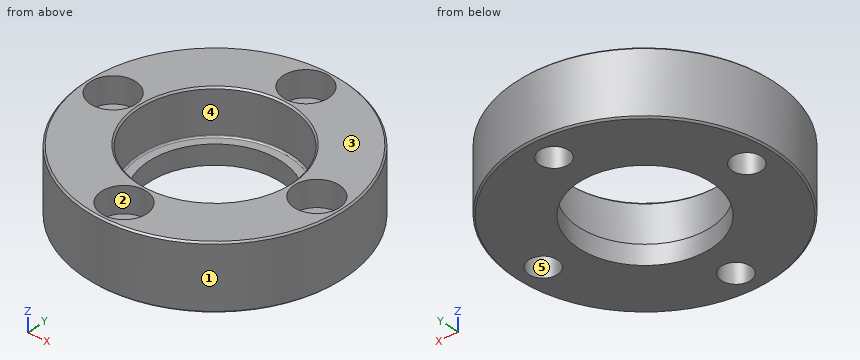
from build123d import *

# Parameters (mm, degrees)
F0_R           = 40
F0_R_2         = 20.5
F1_DEPTH       = 10
F2_R           = 23.5
F3_DEPTH       = 14
F4_R           = 0.5
F5_SIZE        = 0.5
F7_D           = 9
F7_CBORE_D     = 14
F7_CBORE_DEPTH = 8


with BuildPart() as f1:
    # F0 (on Top) → F1 (new body, symmetric)
    with BuildSketch(Plane.XY):
        Circle(F0_R)
        Circle(F0_R_2, mode=Mode.SUBTRACT)
    extrude(amount=F1_DEPTH, both=True)

    # F2 (on face) → F3 (cut)
    with BuildSketch(Plane.XY.offset(10)):
        Circle(F2_R)
    extrude(amount=-F3_DEPTH, mode=Mode.SUBTRACT)

    # F4
    f4_edges = [f1.edges().sort_by_distance(p)[0] for p in [
        (-23.5, 0, -4),
    ]]
    fillet(f4_edges, radius=F4_R)

    # F5
    f5_edges = [f1.edges().sort_by_distance(p)[0] for p in [
        (-23.5, 0, 10),
        (-40, 0, 10),
        (-40, 0, -10),
    ]]
    chamfer(f5_edges, length=F5_SIZE)

    # F7 (through all)
    with Locations(Plane.XY.offset(10)):
        with Locations((0, 31.75), (0, -31.75), (31.75, 0), (-31.75, 0)):
            CounterBoreHole(F7_D / 2, F7_CBORE_D / 2, F7_CBORE_DEPTH)


solid = f1.part
Geometry: final body of the model. Coordinates: model frame, mm. Face numbers are marked on the shaded views. A direction names the side the tool comes from. Round coordinates to 2 decimals unless told otherwise and drop trailing zeros. Order: outer loops, then holes, each group sorted by start corner. A loop starts at its lowest first (then second) coordinate and runs counter-clockwise, first axis right, second up. Notation, with made-up numbers: (55, 7.5) -> (98, 7.5) arc R19 ccw to (98, 24.5) -> close; hole circle Ø7 at (87.25, 7). An arc over 180 degrees is marked (long way). Put each result on its own line as item: value. Start each with the question number.
Q1. First-contact query: pin 1 (11 mm diameter, centred on x = -32, y = 2, fed in from +Z); pin 2 (6 mm diameter, centred on y = 10.5, z = 5.5, fed in from -X); pin 3 (6 mm diameter, centred on x = 24, z = 7, fed in from +Y); pin 4 (7 mm diameter, centred on x = -3, y = -33, fed in from +Z). Flat tips, straight axial feed; report the tip coordinate or a pass-through.
Q2. Reachability of the marked faces 4 and 5 from +Z, -Z, +X, -X, +Y, -Y: full face, straight path, thin tool, end or side. Return the list, or none.
Q3. Section A-A on z = -1.75. Return the cut outline in (x, y), and give its area (3 significant figures).
Q4. Pull-direction query (Y, two-part tool) for the marked faces 1, 2 and 3; classes: +Y half, -Y half, draft (parallel to the pull), parting line (faces both ways), or undercut.
Q5. Section B-B on x = 0. Give the number of separate pieces and of enclosed holes in the cut face, and give its area (3 significant figures).
Q6. Line query: probe 1 along Y at (x, z) = (0, 8); probe 2 along Y at (x, z) = (0, -2.5); probe 3 along X at (y, z) = (6, 6.5). Output: solid intervals per line, ascending.
Q7. Section D-D on z = 4.25. Return the cut outline in (x, y), and give its area (3 significant figures).
Ans:
1. pin 1: stops at z = 10
1. pin 2: stops at x = -39.29
1. pin 3: stops at y = 34.04
1. pin 4: stops at z = 2
2. face 4: +Z
2. face 5: +Z, -Z
3. outline: circle Ø80 at (0, 0); hole circle Ø9 at (-31.75, 0); hole circle Ø47 at (0, 0); hole circle Ø9 at (0, -31.75); hole circle Ø9 at (0, 31.75); hole circle Ø9 at (31.75, 0)
3. area: 3,040 mm2
4. face 1: parting line
4. face 2: undercut
4. face 3: draft
5. separate pieces: 4
5. enclosed holes: 0
5. area: 255 mm2
6. probe 1: y = -40 to -38.75, -24.75 to -23.5, 23.5 to 24.75, 38.75 to 40
6. probe 2: y = -40 to -36.25, -27.25 to -23.5, 23.5 to 27.25, 36.25 to 40
6. probe 3: x = -39.55 to -35.36, -28.14 to -22.72, 22.72 to 28.14, 35.36 to 39.55
7. outline: circle Ø80 at (0, 0); hole circle Ø14 at (-31.75, 0); hole circle Ø47 at (0, 0); hole circle Ø14 at (0, -31.75); hole circle Ø14 at (0, 31.75); hole circle Ø14 at (31.75, 0)
7. area: 2,680 mm2
